Autodesk Inventor part; units mm, degrees
ref_plane "YZ Plane" through (0, 0, 0) normal (1, 0, 0) x (0, 1, 0)
ref_plane "XZ Plane" through (0, 0, 0) normal (0, 1, 0) x (-1, 0, 0)
ref_plane "XY Plane" through (0, 0, 0) normal (0, 0, 1) x (1, 0, 0)
sketch "Эскиз1" plane through (0, 0, 0) normal (0, 0, 1) x (1, 0, 0)
  arc A0 (-21.1675, -5) -> (-19.1116, 10.383) centre (0, 0) ccw
  arc A1 (-18.5893, -5) -> (-16.246, 10.3262) centre (0, 0) ccw
  line L0 (-18.5893, 5) -> (-18.5893, -5) construction
  line L1 (-19.3556, 7.1054) -> (-18.5893, 5)
  line L2 (-18.5893, 5) -> (-16.4242, 6.25)
  line L3 (-16.4242, 6.25) -> (-16.629, 6.8124)
  line L4 (-18.5893, 0) -> (0, 0) construction
  arc A2 (-19.1116, 10.383) -> (-19.3556, 7.1054) centre (-15.5969, 8.4735) ccw
  arc A3 (-16.246, 10.3262) -> (-16.629, 6.8124) centre (-12.8702, 8.1805) ccw
  line L5 (-21.1675, -5) -> (-18.5893, -5)
  point P0 (-19.9352, 8.6978)
  point P1 (-17.2553, 8.5333)
  dimension "d0" = 21.75
  dimension "d1" = 2.5
  dimension "d4" = 10
  dimension "d6" = 30
  dimension "d7" = 100
  dimension "d8" = 2.5
  dimension "d9" = 4
extrude "Выдавливание1" add sketch "Эскиз1" along normal mid plane 1
properties part number "68. Кольцо стопорное подшипника"
Could you check a few things on this model? Use its own coordinates, in mm. A direction names the side the tool comes from. Coordinates: 2 decimals unless noted, no trailing zeros. Order: outer loops, then holes, each group sorted by start corner. A loop starts at its lowest first (then second) coordinate and runs counter-clockwise, first axis right, second up. Notation, with made-up numbers: M 70.5,31.5 L 101.5,31.5 A11 cw 101.5,38.5 Z; hole C 38.5,8.5 d7. An arc over 180 degrees is marked long. Use a Markdown table: item, result. Add a question column.
Q1. Which directions (+Z, -Z, +X, -X, +Y, -Y) give clear straight access to the entire face, cutting with the end or side of a thin tool? Please do faces 4 (the flat face through (-18.98, 6.07, -0.01)), 5 (the flat face through (-17.522, 5.616, -0.007)), 6 (the flat face through (18, -8, -0.5)).
Q2. We'd pull the mould along Y, two halves only. Please class faces 1 (the cylindrical face through (-16.85, 8.59, -0.01)), 2 (the flat face through (18, -8, 0.5)), 3 (the cylindrical face through (21.654, -2.041, -0.007)): pulls with the +Y half, pulls with the -Y half, needs draft (parallel to the pull), parting line crosses it, or undercut.
Q3. I want a section at C-C on y = 13.5. List the corners of the cut face in (x, z) for me.
Q4. I want a section at B-B on x = 15.5. List the corners of the cut face in (y, z) for me, then the cut area to 3 significant figures.
Q5. I'm going to push a flat-ended pin straight in: pin 1 (8 mm diameter, centred on x = -4, y = 16, fed in from -Z). Where does the tip first touch, or does it pass through?
Q6. I want a section at D-D on y = -4. List the corners of the cut face in (x, z) for me, then the cut area to 3 significant figures.
Q7. I want a section at A-A on z = -0.15. List the corners of the cut face in (x, y) for me.
Q8. If I drill on L1, parallel to Y at x = 0.5, z = -0.05; L2, parallel to Y at x = -2, z = 0.15; L3, parallel to X at y = 15, z = 0.4, over which ranges is the centre line in solid material (lowest first)?
Checked values:
| question | item | result |
|---|---|---|
| 1 | face 4 | +Z, -Z, -X |
| 1 | face 5 | +Z, -Z |
| 1 | face 6 | -Z, +X, -X, +Y, -Y |
| 2 | face 1 | undercut |
| 2 | face 2 | needs draft |
| 2 | face 3 | parting line crosses it |
| 3 | outline | M -17.05,-0.5 L -13.72,-0.5 L -13.72,0.5 L -17.05,0.5 Z; M 13.72,-0.5 L 17.05,-0.5 L 17.05,0.5 L 13.72,0.5 Z |
| 4 | outline | M -15.26,-0.5 L -11.42,-0.5 L -11.42,0.5 L -15.26,0.5 Z; M 11.42,-0.5 L 15.26,-0.5 L 15.26,0.5 L 11.42,0.5 Z |
| 4 | area | 7.69 mm² |
| 5 | pin 1 | z = -0.5 |
| 6 | outline | M 18.83,-0.5 L 21.38,-0.5 L 21.38,0.5 L 18.83,0.5 Z |
| 6 | area | 2.55 mm² |
| 7 | outline | M -21.17,-5 A21.75 ccw long -19.11,10.38 A4 ccw -19.36,7.11 L -18.59,5 L -16.42,6.25 L -16.63,6.81 A4 cw -16.25,10.33 A19.25 cw long -18.59,-5 Z |
| 8 | L1 | -21.74 to -19.24, 19.24 to 21.74 |
| 8 | L2 | -21.66 to -19.15, 19.15 to 21.66 |
| 8 | L3 | -15.75 to -12.06, 12.06 to 15.75 |
